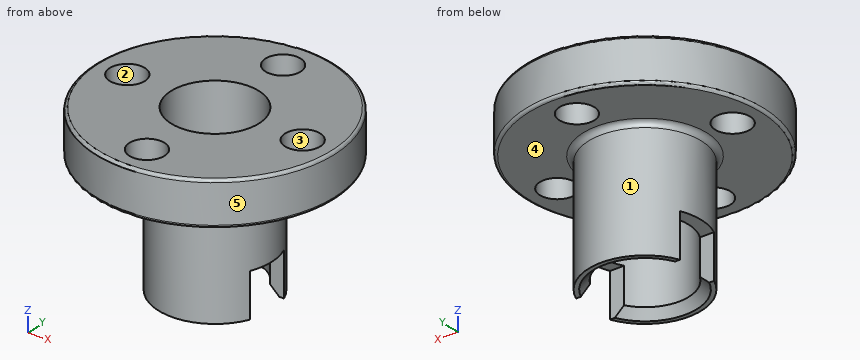
from build123d import *

# Parameters (mm, degrees)
SKETCH2_R          = 4
CUT_EXTRUDE1_DEPTH = 22.483278381
SKETCH3_R          = 1.6
CUT_EXTRUDE2_DEPTH = 19.908496767
SKETCH4_W          = 4
SKETCH4_H          = 4
CUT_EXTRUDE3_DEPTH = 25.496249713
CHAMFER1_SIZE      = 0.75
CHAMFER2_SIZE      = 0.75
FILLET1_R          = 0.5
FILLET2_R          = 0.25


with BuildPart() as part:
    # Sketch1 → Revolve1 (revolve)
    with BuildSketch(Plane(origin=(0, 0, 0), x_dir=(1, 0, 0), z_dir=(0, 1, 0))):
        Polygon((0, 0), (-10.875, 0), (-10.875, 4), (-5.15, 4), (-5.15, 15), (0, 15), align=None)
    revolve(axis=Axis((0, 0, -15), (0, 0, 1)))

    # Sketch2 → Cut-Extrude1 (cut, through all)
    with BuildSketch(Plane(origin=(0, 0, -15), x_dir=(-1, 0, 0), z_dir=(0, 0, -1))):
        Circle(SKETCH2_R)
    extrude(amount=-CUT_EXTRUDE1_DEPTH, mode=Mode.SUBTRACT)

    # Sketch3 → Cut-Extrude2 (cut, through all)
    with BuildSketch(Plane(origin=(0, 0, -4), x_dir=(-1, 0, 0), z_dir=(0, 0, -1))):
        with Locations((0, 8)):
            Circle(SKETCH3_R)
        with Locations((8, 0)):
            Circle(SKETCH3_R)
        with Locations((0, -8)):
            Circle(SKETCH3_R)
        with Locations((-8, 0)):
            Circle(SKETCH3_R)
    extrude(amount=-CUT_EXTRUDE2_DEPTH, mode=Mode.SUBTRACT)

    # Sketch4 → Cut-Extrude3 (cut, through all)
    with BuildSketch(Plane(origin=(5.15, 0, 0), x_dir=(0, 0, -1), z_dir=(1, 0, 0))):
        with Locations((13, 0)):
            Rectangle(SKETCH4_W, SKETCH4_H)
    extrude(amount=-CUT_EXTRUDE3_DEPTH, mode=Mode.SUBTRACT)

    # Chamfer1
    chamfer1_edges = [part.edges().sort_by_distance(p)[0] for p in [
        (0, 4, -15),
    ]]
    chamfer(chamfer1_edges, length=CHAMFER1_SIZE)

    # Chamfer2
    chamfer2_edges = [part.edges().sort_by_distance(p)[0] for p in [
        (0, -4, -15),
    ]]
    chamfer(chamfer2_edges, length=CHAMFER2_SIZE)

    # Fillet1
    fillet1_edges = [part.edges().sort_by_distance(p)[0] for p in [
        (5.15, 0, -4),
    ]]
    fillet(fillet1_edges, radius=FILLET1_R)

    # Fillet2
    fillet2_edges = [part.edges().sort_by_distance(p)[0] for p in [
        (10.875, 0, -4),
        (10.875, 0, 0),
    ]]
    fillet(fillet2_edges, radius=FILLET2_R)


solid = part.part
The listing builds one solid part. Answer for the finished solid, in the listing's coordinates (mm). Face numbers are marked on the shaded views. A direction names the side the tool comes from. Coordinates: 2 decimals unless noted, no trailing zeros. Loops run counter-clockwise (first coordinate to the right, second up) from the corner with the lowest first, then second, coordinate; pieces in that order, holes last.
1) Flat-ended cylindrical pins translate along their axes: pin 1 Ø3.5 at (x, y) = (8, 0) entering from -Z; pin 2 Ø1.4 at (x, z) = (-4.5, -13.5) entering from +Y; pin 3 Ø2.5 at (x, y) = (0, -8) entering from -Z; pin 4 Ø0.6 at (x, z) = (-4, -12.5) entering from -Y. Find the tip coordinate at first contact, or state that the pin passes through.
2) Determine the mould class of the marked faces 3, 4 and 5 for opening direction Y: pulls with the +Y half, pulls with the -Y half, needs draft (parallel to the pull), parting line crosses it, or undercut.
3) Find section D-D on z = -9.5. Write down the section's boundary in (x, y), then the cut area to 3 significant figures.
4) Find section C-C on z = -3.25. Write down the section's boundary in (x, y) (3 decimals), then the cut area to 3 significant figures.
5) Find the intervals of material crossed by L1, parallel to Y at x = 0, z = -3 (3 decimals); L2, parallel to X at y = -1.25, z = -2.25; L3, parallel to Y at x = 0, z = -8.25, in increasing order.
6) A tool of negligible diameter and unlimited length cuts with its end or side. For the marked faces 1 and 2, from which of +Z, -Z, +X, -X, +Y, -Y can it reach the whole face along a straight path? Write none if from no direction.
7) Find section B-B on x = 0. Write down the section's boundary in (y, z) (3 decimals), then the cut area to 3 significant figures.
8) Find section A-A on z = -13.75. Write down the section's boundary in (x, y).
Values:
1. pin 1: stops at z = -4
1. pin 2: stops at y = 3.48
1. pin 3: passes through
1. pin 4: stops at y = -3.58
2. face 3: undercut
2. face 4: needs draft
2. face 5: parting line crosses it
3. outline: circle Ø10.3 at (0, 0); hole circle Ø8 at (0, 0)
3. area: 33.1 mm2
4. outline: circle Ø21.75 at (0, 0); hole circle Ø3.2 at (-8, 0); hole circle Ø8 at (0, 0); hole circle Ø3.2 at (0, -8); hole circle Ø3.2 at (0, 8); hole circle Ø3.2 at (8, 0)
4. area: 289 mm2
5. L1: y = -10.875 to -9.6, -6.4 to -4, 4 to 6.4, 9.6 to 10.875
5. L2: x = -10.8 to -9, -7 to -3.8, 3.8 to 7, 9 to 10.8
5. L3: y = -5.15 to -4, 4 to 5.15
6. face 1: -Z
6. face 2: +Z, -Z
7. outline: (-10.875, -3.75) arc R0.25 ccw to (-10.625, -4) - (-9.6, -4) - (-9.6, 0) - (-10.625, 0) arc R0.25 ccw to (-10.875, -0.25) - close; (-6.4, -4) - (-5.65, -4) arc R0.5 cw to (-5.15, -4.5) - (-5.15, -15) - (-4.75, -15) - (-4, -14.25) - (-4, 0) - (-6.4, 0) - close; (4, -14.25) - (4.75, -15) - (5.15, -15) - (5.15, -4.5) arc R0.5 cw to (5.65, -4) - (6.4, -4) - (6.4, 0) - (4, 0) - close; (9.6, -4) - (10.625, -4) arc R0.25 ccw to (10.875, -3.75) - (10.875, -0.25) arc R0.25 ccw to (10.625, 0) - (9.6, 0) - close
7. area: 54.2 mm2
8. outline: (-4.75, -2) arc R5.15 ccw to (4.75, -2) - (3.46, -2) arc R4 cw to (-3.46, -2) - close; (-4.75, 2) - (-3.46, 2) arc R4 cw to (3.46, 2) - (4.75, 2) arc R5.15 ccw to start
